CAD build for the part. Positions are in the model's coordinates, mm. Give positions to 0.01 mm unless a question says otherwise; leave off trailing zeros. Loops run counter-clockwise (first coordinate to the right, second up) from the corner with the lowest first, then second, coordinate; pieces in that order, holes last.
Item 1: Saw through at B-B on z = 0. Give the cut face in (x, y).
Item 2: Drop a flat-ended pin along its axis: P1, Ø1.5, axis at y = 0.5, z = 2.5, coming from the +X side. Give the stop position or say it passes through.
Item 3: Saw through at C-C on x = 59.7. Give the cut face in (y, z).
Item 4: Mould opens along Z. For faces 1 (the cylindrical face through (0.37, 1.48, 1.66)), 2 (the flat face through (48, 0, 0)), 3 (the cylindrical face through (-4, 1, 0)) say: released by +Z, released by -Z, zero draft, split by the parting line, or undercut.
Item 5: Saw through at A-A on y = 2.45. Give the cut face in (x, z).
Item 6: Probe probe 1 along Z at (x, y) = (59.7, 2.15); probe 2 along X at (y, z) = (1.1, 0.25); probe 3 along Z at (x, y) = (0, 2.25). List the from-to ranges inside material, lowest first.
from build123d import *

# Parameters (mm, degrees)
BOSS_EXTRUDE1_DEPTH  = 3
M3_CLEARANCE_HOLE1_D = 3.4
M2_CLEARANCE_HOLE1_D = 2.4


with BuildPart() as part:
    # Sketch1 → Boss-Extrude1 (new body)
    with BuildSketch(Plane(origin=(0, 0, 0), x_dir=(1, 0, 0), z_dir=(0, 1, 0))):
        with BuildLine():
            Line((0, 4), (95, 4))
            ThreePointArc((95, 4), (99, 0), (95, -4))
            Line((95, -4), (0, -4))
            ThreePointArc((0, -4), (-4, 0), (0, 4))
        make_face()
    extrude(amount=BOSS_EXTRUDE1_DEPTH)

    # M3 Clearance Hole1 (through all)
    with Locations(Plane(origin=(0, 3, 0), x_dir=(1, 0, 0), z_dir=(0, 1, 0))):
        with Locations((95, 0), (0, 0)):
            Hole(M3_CLEARANCE_HOLE1_D / 2)

    # M2 Clearance Hole1 (through all)
    with Locations(Plane(origin=(0, 3, 0), x_dir=(1, 0, 0), z_dir=(0, 1, 0))):
        with Locations((59.7, 0), (35.3, 0)):
            Hole(M2_CLEARANCE_HOLE1_D / 2)


solid = part.part
Results below:
1. outline: (-4, 0) - (-1.7, 0) - (-1.7, 3) - (-4, 3) - close; (1.7, 0) - (34.1, 0) - (34.1, 3) - (1.7, 3) - close; (36.5, 0) - (58.5, 0) - (58.5, 3) - (36.5, 3) - close; (60.9, 0) - (93.3, 0) - (93.3, 3) - (60.9, 3) - close; (96.7, 0) - (99, 0) - (99, 3) - (96.7, 3) - close
2. P1: stops at x = 98.6
3. outline: (0, -4) - (3, -4) - (3, -1.2) - (0, -1.2) - close; (0, 1.2) - (3, 1.2) - (3, 4) - (0, 4) - close
4. face 1: undercut
4. face 2: zero draft
4. face 3: split by the parting line
5. outline: (0, -4) - (95, -4) arc R4 ccw to (95, 4) - (0, 4) arc R4 ccw to start; hole circle Ø3.4 at (0, 0); hole circle Ø2.4 at (35.3, 0); hole circle Ø2.4 at (59.7, 0); hole circle Ø3.4 at (95, 0)
6. probe 1: z = -4 to -1.2, 1.2 to 4
6. probe 2: x = -3.99 to -1.68, 1.68 to 34.13, 36.47 to 58.53, 60.87 to 93.32, 96.68 to 98.99
6. probe 3: z = -4 to -1.7, 1.7 to 4
